Verification items for the finished model (mm, model axes). A direction names the side the tool comes from. Coordinates: 2 decimals unless noted, no trailing zeros. Write each loop counter-clockwise with the first axis right and the second up, starting at its lowest first coordinate (ties: lowest second). Pieces come first, ordered by that corner, then holes. Notation, with made-up numbers: (-13, -17.75) -> (5, -17.75) arc R16 cw to (5, -3.75) -> close; hole circle Ø5 at (-37.5, -39). An arc over 180 degrees is marked (long way). Write item = value, one per line. Start each with the question number.
(1) Material ranges on probe 1 along Z at (x, y) = (-16.5, 193.5) (3 decimals); probe 2 along X at (y, z) = (894.5, 7.75) (3 decimals); probe 3 along X at (y, z) = (952.5, -11.6), recorded low to high. Write a range as [from, to].
(2) Section check A-A (y = 664). Record the cut outline in (x, z) (3 decimals).
(3) Set-up check for faces 1 (the face through (0, 526, -12.7)), 2 (the face through (-22.225, 526, 0)): record each of +Z, -Z, +X, -X, +Y, -Y from which the full face is reachable in a straight line by a thin tool's end or side.
(4) Mould release check, pull along X, two halves, no side actions. Record for faces 3 (the face through (-25.4, 526, 0)), 4 (the face through (-1.86, 1055.566, 11.135)), 5 (the face through (0, 526, 9.525)), 6 (the face through (25.4, 526, 0)): released by +X, released by -X, zero draft, split by the parting line, or undercut.
```python
from build123d import *

# Parameters (mm, degrees)
SKETCH1_W                        = 50.8
SKETCH1_H                        = 25.4
SKETCH1_W_2                      = 44.45
SKETCH1_H_2                      = 19.05
BOSS_EXTRUDE1_DEPTH              = 1066.8
SKETCH2_R                        = 14.2875
CUT_EXTRUDE1_DEPTH               = 1068.404590584
SKETCH3_R                        = 3.3734375
CUT_EXTRUDE2_DEPTH               = 1068.404590584
SKETCH4_R                        = 3.3734375
CUT_EXTRUDE3_DEPTH               = 1068.404590584
SKETCH5_R                        = 3.3734375
CUT_EXTRUDE4_DEPTH               = 1068.404590584
F_13_64_0_20313_DIAMETER_HOLE1_D = 5.159502
F_13_64_0_20313_DIAMETER_HOLE2_D = 5.159502
SKETCH10_R                       = 3.3734375
CUT_EXTRUDE5_DEPTH               = 1068.404590584
SKETCH11_R                       = 3.3734375
CUT_EXTRUDE6_DEPTH               = 1068.404590584


with BuildPart() as part:
    # Sketch1 → Boss-Extrude1 (new body)
    with BuildSketch(Plane(origin=(0, 0, 0), x_dir=(1, 0, 0), z_dir=(0, 1, 0))):
        Rectangle(SKETCH1_W, SKETCH1_H)
        Rectangle(SKETCH1_W_2, SKETCH1_H_2, mode=Mode.SUBTRACT)
    extrude(amount=BOSS_EXTRUDE1_DEPTH)

    # Sketch2 → Cut-Extrude1 (cut, through all)
    with BuildSketch(Plane.XY.offset(12.7)):
        with Locations((0, 1041.4)):
            Circle(SKETCH2_R)
    extrude(amount=-CUT_EXTRUDE1_DEPTH, mode=Mode.SUBTRACT)

    # Sketch3 → Cut-Extrude2 (cut, through all)
    with BuildSketch(Plane.XY.offset(12.7)):
        with Locations((0, 313.436)):
            Circle(SKETCH3_R)
    extrude(amount=-CUT_EXTRUDE2_DEPTH, mode=Mode.SUBTRACT)

    # Sketch4 → Cut-Extrude3 (cut, through all)
    with BuildSketch(Plane.XY.offset(12.7)):
        with Locations((0, 351.536)):
            Circle(SKETCH4_R)
    extrude(amount=-CUT_EXTRUDE3_DEPTH, mode=Mode.SUBTRACT)

    # Sketch5 → Cut-Extrude4 (cut, through all)
    with BuildSketch(Plane.XY.offset(12.7)):
        with Locations((0, 12.7)):
            Circle(SKETCH5_R)
        with Locations((0, 38.1)):
            Circle(SKETCH5_R)
    extrude(amount=-CUT_EXTRUDE4_DEPTH, mode=Mode.SUBTRACT)

    # 13/64 (0.20313) Diameter Hole1 (through all)
    with Locations(Plane(origin=(0, 0, -12.7), x_dir=(-1, 0, 0), z_dir=(0, 0, -1))):
        with Locations((-1.269999999, 519.585439927), (-1.269999999, 494.185439927)):
            Hole(F_13_64_0_20313_DIAMETER_HOLE1_D / 2)

    # 13/64 (0.20313) Diameter Hole2 (through all)
    with Locations(Plane(origin=(0, 0, -12.7), x_dir=(-1, 0, 0), z_dir=(0, 0, -1))):
        with Locations((0, 977.9), (0, 952.5), (0, 927.1)):
            Hole(F_13_64_0_20313_DIAMETER_HOLE2_D / 2)

    # Sketch10 → Cut-Extrude5 (cut, through all)
    with BuildSketch(Plane(origin=(0, 0, -12.7), x_dir=(-1, 0, 0), z_dir=(0, 0, -1))):
        with Locations((0, 76.2)):
            Circle(SKETCH10_R)
    extrude(amount=-CUT_EXTRUDE5_DEPTH, mode=Mode.SUBTRACT)

    # Sketch11 → Cut-Extrude6 (cut, through all)
    with BuildSketch(Plane(origin=(0, 0, -12.7), x_dir=(-1, 0, 0), z_dir=(0, 0, -1))):
        with Locations((-17.779998161, 155.17537)):
            Circle(SKETCH11_R)
        with Locations((17.780001839, 155.17537)):
            Circle(SKETCH11_R)
    extrude(amount=-CUT_EXTRUDE6_DEPTH, mode=Mode.SUBTRACT)


solid = part.part
```
Response:
q1.probe_1 = [-12.7, -9.525], [9.525, 12.7]
q1.probe_2 = [-25.4, -22.225], [22.225, 25.4]
q1.probe_3 = [-25.4, -2.58], [2.58, 25.4]
q2.outline = (-25.4, -12.7) -> (25.4, -12.7) -> (25.4, 12.7) -> (-25.4, 12.7) -> close; hole (-22.225, -9.525) -> (22.225, -9.525) -> (22.225, 9.525) -> (-22.225, 9.525) -> close
q3.face_1 = -Z, +X, -X, +Y, -Y
q3.face_2 = +Y, -Y
q4.face_3 = released by -X
q4.face_4 = undercut
q4.face_5 = undercut
q4.face_6 = released by +X
